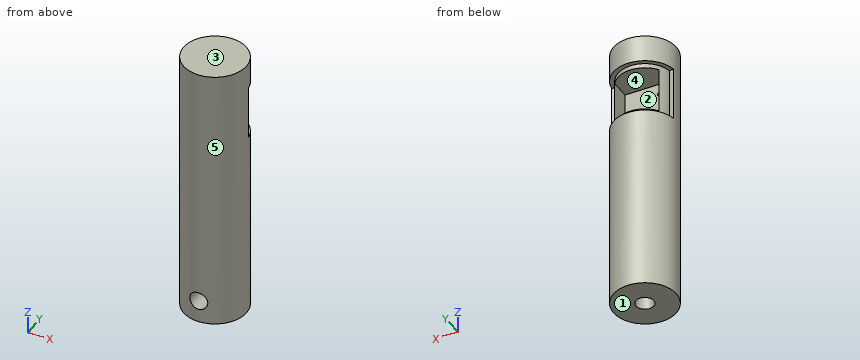
```python
from build123d import *

# Parameters (mm, degrees)
SKETCH2_R           = 22.225
BOSS_EXTRUDE1_DEPTH = 190.5
SKETCH3_R           = 6.35
CUT_EXTRUDE1_DEPTH  = 139.7
WRAP1_SECTION_W     = 3.175
WRAP1_SECTION_H     = 38.1
WRAP1_ANGLE         = 163.70222718
SKETCH6_W           = 31.75
SKETCH6_H           = 31.75
CUT_EXTRUDE2_DEPTH  = 25.4
SKETCH7_R           = 1.190625
CUT_EXTRUDE3_DEPTH  = 31.75
SKETCH8_R           = 6.35
CUT_EXTRUDE4_DEPTH  = 22.225


with BuildPart() as part:
    # Sketch2 → Boss-Extrude1 (new body)
    with BuildSketch(Plane.XY):
        Circle(SKETCH2_R)
    extrude(amount=-BOSS_EXTRUDE1_DEPTH)

    # Sketch3 → Cut-Extrude1 (cut)
    with BuildSketch(Plane(origin=(0, 0, -190.5), x_dir=(-1, 0, 0), z_dir=(0, 0, -1))):
        Circle(SKETCH3_R)
    extrude(amount=-CUT_EXTRUDE1_DEPTH, mode=Mode.SUBTRACT)

    # Wrap1 section (on wrap section) → Wrap1 (revolve, cut)
    with BuildSketch(Plane(origin=(0, 0, 0), x_dir=(0.9899030763721239, 0.14174589725634046, 0), z_dir=(0.14174589725634046, -0.9899030763721239, 0))):
        with Locations((20.6375, -38.1)):
            Rectangle(WRAP1_SECTION_W, WRAP1_SECTION_H)
    revolve(axis=Axis((0, 0, 0), (0, 0, 1)), revolution_arc=WRAP1_ANGLE, mode=Mode.SUBTRACT)

    # Sketch6 → Cut-Extrude2 (cut)
    with BuildSketch(Plane(origin=(0, 22.225, 0), x_dir=(1, 0, 0), z_dir=(0, 1, 0))):
        with Locations((0, 38.1)):
            Rectangle(SKETCH6_W, SKETCH6_H)
    extrude(amount=-CUT_EXTRUDE2_DEPTH, mode=Mode.SUBTRACT)

    # Sketch7 → Cut-Extrude3 (cut)
    with BuildSketch(Plane(origin=(0, 22.225, 0), x_dir=(1, 0, 0), z_dir=(0, 1, 0))):
        with Locations(Location((-8.255, 29.845, 0), (0, 0, 270))):
            Circle(SKETCH7_R)
        with Locations(Location((8.255, 46.355, 0), (0, 0, 270))):
            Circle(SKETCH7_R)
    extrude(amount=-CUT_EXTRUDE3_DEPTH, mode=Mode.SUBTRACT)

    # Sketch8 → Cut-Extrude4 (cut)
    with BuildSketch(Plane(origin=(0, -22.225, 0), x_dir=(-1, 0, 0), z_dir=(0, -1, 0))):
        with Locations(Location((0, 174.625, 0), (0, 0, 90))):
            Circle(SKETCH8_R)
    extrude(amount=-CUT_EXTRUDE4_DEPTH, mode=Mode.SUBTRACT)


solid = part.part
```
Source: CAD feature listing. Evaluate the final solid. Frame: model axes, mm. Face numbers are marked on the shaded views. A direction names the side the tool comes from. Round coordinates to 2 decimals unless told otherwise and drop trailing zeros. Loops run counter-clockwise (first coordinate to the right, second up) from the corner with the lowest first, then second, coordinate; pieces in that order, holes last. Notation, with made-up numbers: M -7.5,37 L 28.5,37 A17 cw 28.5,61 Z; hole C 36.25,54 d9. An arc over 180 degrees is marked long. Use a Markdown table: item, result. Add a question column.
1. Cut plane C-C, the plane z = -125. Output: boundary loops of the cut face in (x, y) (3 decimals).
2. Pull-direction query (Z, two-part tool) for the marked faces 1, 2 and 3; classes: +Z half, -Z half, draft (parallel to the pull), parting line (faces both ways), or undercut.
3. Cut plane A-A, the plane x = 0. Output: boundary loops of the cut face in (y, z) (3 decimals).
4. Cut plane B-B, the plane y = 8. Output: boundary loops of the cut face in (x, z) (3 decimals).
5. Contact query for flat-ended pins moving along their axis: pin 1 (10 mm diameter, centred on y = -15, z = -163.5, fed in from +X); pin 2 (2.5 mm diameter, centred on x = -8, z = -30, fed in from +Y) (3 decimals); pin 3 (7 mm diameter, centred on y = 4.5, z = -37.5, fed in from +X). Output: stop coordinate, or through.
6. Ray query, line 1 along Z through (x, y) = (19, 8); line 2 along Z through (x, y) = (12.5, 4) (3 decimals); line 3 along X through (y, z) = (0.5, -167). Return the intervals inside material, ascending. Write a range as [from, to].
7. Cut plane D-D, the plane y = -16.5. Output: boundary loops of the cut face in (x, z) (3 decimals).
8. Set-up query: the marked faces 4 and 5. Return all of +Z, -Z, +X, -X, +Y, -Y with unobstructed straight access to the full face (end or side cutting, diameter ignored); none if empty.
Solution:
| question | item | result |
|---|---|---|
| 1 | outline | C 0,0 d44.45; hole C 0,0 d12.7 |
| 2 | face 1 | -Z half |
| 2 | face 2 | undercut |
| 2 | face 3 | +Z half |
| 3 | outline | M -22.225,-190.5 L -6.35,-190.5 L -6.35,-180.975 L -22.225,-180.975 Z; M -22.225,-168.275 L -6.35,-168.275 L -6.35,-50.8 L -3.175,-50.8 L -3.175,-22.225 L 19.05,-22.225 L 19.05,-19.05 L 22.225,-19.05 L 22.225,0 L -22.225,0 Z; M 6.35,-190.5 L 22.225,-190.5 L 22.225,-57.15 L 19.05,-57.15 L 19.05,-53.975 L 6.35,-53.975 Z |
| 4 | outline | M -20.735,-190.5 L 20.735,-190.5 L 20.735,-57.15 L 17.289,-57.15 L 17.289,-19.05 L 20.735,-19.05 L 20.735,0 L -20.735,0 L -20.735,-19.05 L -17.289,-19.05 L -17.289,-57.15 L -20.735,-57.15 Z; hole M -15.875,-53.975 L 15.875,-53.975 L 15.875,-22.225 L -15.875,-22.225 Z |
| 5 | pin 1 | stops at x = 19.85 |
| 5 | pin 2 | stops at y = -3.175 |
| 5 | pin 3 | stops at x = 22.2 |
| 6 | line 1 | z = [-190.5, -57.15], [-19.05, 0] |
| 6 | line 2 | z = [-190.5, -53.975], [-22.225, 0] |
| 6 | line 3 | x = [-22.22, -6.33], [6.33, 22.22] |
| 7 | outline | M -14.89,-190.5 L 14.89,-190.5 L 14.89,0 L -14.89,0 Z; hole C 0,-174.625 d12.7 |
| 8 | face 4 | +Y |
| 8 | face 5 | +Z, -Z |
